```python
from build123d import *
from build123d.topology import SkipClean

# Parameters (mm, degrees)
BOSS_EXTRUDE1_DEPTH     = 3
CROQUIS1_W              = 50.575264902
CROQUIS1_H              = 364.883290788
CROQUIS1_W_2            = 121.011581191
CROQUIS1_H_2            = 356.31671178
CORTAR_EXTRUIR1_DEPTH   = 10
CROQUIS2_W              = 390
CROQUIS2_H              = 250
SALIENTE_EXTRUIR1_DEPTH = 3
CROQUIS3_W              = 60
CROQUIS3_H              = 30
CORTAR_EXTRUIR3_DEPTH   = 3
CROQUIS4_W              = 90
CROQUIS4_H              = 3
SALIENTE_EXTRUIR2_DEPTH = 3
CROQUIS5_W              = 30
CROQUIS5_H              = 30
CORTAR_EXTRUIR4_DEPTH   = 3
CROQUIS6_W              = 30
CROQUIS6_H              = 38.5
CORTAR_EXTRUIR5_DEPTH   = 3
CROQUIS7_W              = 38.5
CROQUIS7_H              = 30
CORTAR_EXTRUIR6_DEPTH   = 3
CROQUIS8_W              = 137
CROQUIS8_H              = 0.25
CORTAR_EXTRUIR7_DEPTH   = 3
CROQUIS9_W              = 0.25
CROQUIS9_H              = 68.25
CORTAR_EXTRUIR8_DEPTH   = 3
CORTAR_EXTRUIR9_DEPTH   = 3
SALIENTE_EXTRUIR3_DEPTH = 3
CROQUIS12_R             = 4
CORTAR_EXTRUIR10_DEPTH  = 3
CROQUIS13_R             = 4.25
CROQUIS13_R_2           = 3.25
SALIENTE_EXTRUIR4_DEPTH = 3
CROQUIS14_R             = 4.25
CORTAR_EXTRUIR11_DEPTH  = 3
CROQUIS15_R             = 4.25
CORTAR_EXTRUIR12_DEPTH  = 25
SALIENTE_EXTRUIR5_DEPTH = 3
CROQUIS17_R             = 1.5
CORTAR_EXTRUIR13_DEPTH  = 10
CROQUIS18_R             = 1.5
CORTAR_EXTRUIR14_DEPTH  = 30
CROQUIS19_R             = 1.5
SALIENTE_EXTRUIR6_DEPTH = 3
CROQUIS21_R             = 1.5
CORTAR_EXTRUIR15_DEPTH  = 3
SALIENTE_EXTRUIR7_DEPTH = 3
CORTAR_EXTRUIR17_DEPTH  = 10
CORTAR_EXTRUIR18_DEPTH  = 10


with BuildPart() as part:
    # Sketch1 → Boss-Extrude1 (new body)
    with BuildSketch(Plane.XY):
        Polygon((0, 0), (403.39, 0), (403.39, 241), (274.41, 359.5), (128.98, 359.5), (0, 241), align=None)
        Polygon((216.695, 223), (246.695, 223), (246.695, 253), (156.695, 253), (156.695, 223), (186.695, 223), (186.695, 219.825), (216.695, 219.825), align=None, mode=Mode.SUBTRACT)
    extrude(amount=BOSS_EXTRUDE1_DEPTH)

    # Croquis1 → Cortar-Extruir1 (cut)
    with BuildSketch(Plane.XY.offset(3)):
        with Locations((-18.592632451, 182.441645394)):
            Rectangle(CROQUIS1_W, CROQUIS1_H)
        with Locations((457.200790596, 178.15835589)):
            Rectangle(CROQUIS1_W_2, CROQUIS1_H_2)
    extrude(amount=-CORTAR_EXTRUIR1_DEPTH, mode=Mode.SUBTRACT)

    # Croquis2 → Saliente-Extruir1 (add)
    with BuildSketch(Plane.XY.offset(3)):
        with Locations((201.695, 125)):
            Rectangle(CROQUIS2_W, CROQUIS2_H)
    extrude(amount=-SALIENTE_EXTRUIR1_DEPTH)

    # Croquis3 → Cortar-Extruir3 (cut)
    with BuildSketch(Plane.XY.offset(3)):
        with Locations((201.695, 235)):
            Rectangle(CROQUIS3_W, CROQUIS3_H)
    extrude(amount=-CORTAR_EXTRUIR3_DEPTH, mode=Mode.SUBTRACT)

    # Croquis4 → Saliente-Extruir2 (add)
    with BuildSketch(Plane.XY.offset(3)):
        with Locations((201.695, 251.5)):
            Rectangle(CROQUIS4_W, CROQUIS4_H)
    extrude(amount=-SALIENTE_EXTRUIR2_DEPTH)

    # Croquis5 → Cortar-Extruir4 (cut)
    with BuildSketch(Plane.XY.offset(3)):
        with Locations((201.695, 205)):
            Rectangle(CROQUIS5_W, CROQUIS5_H)
    extrude(amount=-CORTAR_EXTRUIR4_DEPTH, mode=Mode.SUBTRACT)

    # Croquis6 → Cortar-Extruir5 (cut)
    with BuildSketch(Plane.XY.offset(3)):
        with Locations((201.695, 170.75)):
            Rectangle(CROQUIS6_W, CROQUIS6_H)
    extrude(amount=-CORTAR_EXTRUIR5_DEPTH, mode=Mode.SUBTRACT)

    # Croquis7 → Cortar-Extruir6 (cut)
    with BuildSketch(Plane.XY.offset(3)):
        with Locations((152.445, 235)):
            Rectangle(CROQUIS7_W, CROQUIS7_H)
        with Locations((250.945, 235)):
            Rectangle(CROQUIS7_W, CROQUIS7_H)
    extrude(amount=-CORTAR_EXTRUIR6_DEPTH, mode=Mode.SUBTRACT)

    # Croquis8 → Cortar-Extruir7 (cut)
    with BuildSketch(Plane.XY.offset(3)):
        with Locations((201.695, 250.125)):
            Rectangle(CROQUIS8_W, CROQUIS8_H)
        with Locations((201.695, 219.875)):
            Rectangle(CROQUIS8_W, CROQUIS8_H)
    extrude(amount=-CORTAR_EXTRUIR7_DEPTH, mode=Mode.SUBTRACT)

    # Croquis9 → Cortar-Extruir8 (cut)
    with BuildSketch(Plane.XY.offset(3)):
        with Locations((186.57, 185.625)):
            Rectangle(CROQUIS9_W, CROQUIS9_H)
        with Locations((216.82, 185.625)):
            Rectangle(CROQUIS9_W, CROQUIS9_H)
    extrude(amount=-CORTAR_EXTRUIR8_DEPTH, mode=Mode.SUBTRACT)

    # Croquis10 → Cortar-Extruir9 (cut)
    with BuildSketch(Plane.XY.offset(3)):
        Polygon((136.695, 348.165217873), (266.695, 348.165217873), (396.695, 250), (402.242964747, 389.308105161), (24.251899655, 412.117910813), (6.695, 250), align=None)
    extrude(amount=-CORTAR_EXTRUIR9_DEPTH, mode=Mode.SUBTRACT)

    # Croquis11 → Saliente-Extruir3 (add)
    with BuildSketch(Plane.XY.offset(3)):
        Polygon((51.733112384, 284.009047037), (6.695, 250), (31.650370126, 216.951653685), align=None)
        Polygon((347.889102287, 286.854166019), (396.695, 250), (356.623353442, 225.729213199), align=None)
    extrude(amount=-SALIENTE_EXTRUIR3_DEPTH)

    # Croquis12 → Cortar-Extruir10 (cut)
    with BuildSketch(Plane.XY.offset(3)):
        with Locations((21.695, 15)):
            Circle(CROQUIS12_R)
        with Locations((381.695, 15)):
            Circle(CROQUIS12_R)
        with Locations((51.695, 235)):
            Circle(CROQUIS12_R)
        with Locations((351.695, 235)):
            Circle(CROQUIS12_R)
    extrude(amount=-CORTAR_EXTRUIR10_DEPTH, mode=Mode.SUBTRACT)

    # Croquis13 → Saliente-Extruir4 (add)
    # profile 1 of 2: a face of its own
    with BuildSketch(Plane.XY.offset(3)):
        with Locations((51.695, 235)):
            Circle(CROQUIS13_R)
        with Locations((51.695, 235)):
            Circle(CROQUIS13_R_2, mode=Mode.SUBTRACT)
    # profile 2 of 2: a face of its own
    with BuildSketch(Plane.XY.offset(3)):
        with Locations((351.695, 235)):
            Circle(CROQUIS13_R)
        with Locations((351.695, 235)):
            Circle(CROQUIS13_R_2, mode=Mode.SUBTRACT)
    extrude(amount=-SALIENTE_EXTRUIR4_DEPTH)

    # Croquis14 → Cortar-Extruir11 (cut)
    with BuildSketch(Plane.XY.offset(3)):
        with Locations((201.695, 35)):
            Circle(CROQUIS14_R)
        with Locations((201.695, 123)):
            Circle(CROQUIS14_R)
    extrude(amount=-CORTAR_EXTRUIR11_DEPTH, mode=Mode.SUBTRACT)

    # Croquis15 → Cortar-Extruir12 (cut)
    with BuildSketch(Plane.XY.offset(3)):
        with Locations((201.695, 38)):
            Circle(CROQUIS15_R)
    extrude(amount=-CORTAR_EXTRUIR12_DEPTH, mode=Mode.SUBTRACT)

    # Croquis16 → Saliente-Extruir5 (add)
    with BuildSketch(Plane.XY.offset(3)):
        with BuildLine():
            ThreePointArc((205.67149343, 36.5), (201.695, 33.75), (197.71850657, 36.5))
            ThreePointArc((197.71850657, 36.5), (200.9326343, 30.818935717), (205.945, 35))
            ThreePointArc((205.945, 35), (205.876064283, 35.7623657), (205.67149343, 36.5))
        make_face()
    extrude(amount=-SALIENTE_EXTRUIR5_DEPTH)

    # Croquis17 → Cortar-Extruir13 (cut)
    with BuildSketch(Plane.XY.offset(3)):
        with Locations((146.568722662, 341.065217873)):
            Circle(CROQUIS17_R)
        with Locations((254.977292633, 341.065217873)):
            Circle(CROQUIS17_R)
        with Locations((134.589248293, 337.678282679)):
            Circle(CROQUIS17_R)
        with Locations((31.642655291, 259.941553977)):
            Circle(CROQUIS17_R)
        with Locations((268.800751707, 337.678282679)):
            Circle(CROQUIS17_R)
        with Locations((371.747344709, 259.941553977)):
            Circle(CROQUIS17_R)
    extrude(amount=-CORTAR_EXTRUIR13_DEPTH, mode=Mode.SUBTRACT)

    # Croquis18 → Cortar-Extruir14 (cut)
    with BuildSketch(Plane.XY.offset(3)):
        with Locations((144.695, 341.065217873)):
            Circle(CROQUIS18_R)
        with Locations((258.695, 341.065217873)):
            Circle(CROQUIS18_R)
    extrude(amount=-CORTAR_EXTRUIR14_DEPTH, mode=Mode.SUBTRACT)

    # Croquis19 → Saliente-Extruir6 (add)
    with BuildSketch(Plane.XY.offset(3)):
        with BuildLine():
            ThreePointArc((145.631861331, 339.893769689), (145.068722662, 341.065217873), (145.631861331, 342.236666056))
            ThreePointArc((145.631861331, 342.236666056), (143.195, 341.065217873), (145.631861331, 339.893769689))
        make_face()
        with Locations((254.977292633, 341.065217873)):
            Circle(CROQUIS19_R)
    extrude(amount=-SALIENTE_EXTRUIR6_DEPTH)

    # Croquis21 → Cortar-Extruir15 (cut)
    with BuildSketch(Plane.XY.offset(3)):
        with Locations((144.695, 341.065217873)):
            Circle(CROQUIS21_R)
    extrude(amount=-CORTAR_EXTRUIR15_DEPTH, mode=Mode.SUBTRACT)

    # Croquis22 → Saliente-Extruir7 (add)
    with BuildSketch(Plane.XY.offset(3)):
        with BuildLine():
            ThreePointArc((145.631861331, 342.236666056), (146.046904582, 341.715105557), (146.195, 341.065217873))
            ThreePointArc((146.195, 341.065217873), (146.046904582, 340.415330189), (145.631861331, 339.893769689))
            ThreePointArc((145.631861331, 339.893769689), (147.218610346, 339.713313291), (148.068722662, 341.065217873))
            ThreePointArc((148.068722662, 341.065217873), (147.218610346, 342.417122454), (145.631861331, 342.236666056))
        make_face()
    extrude(amount=-SALIENTE_EXTRUIR7_DEPTH)

    # Croquis23 → Cortar-Extruir17 (cut)
    with BuildSketch(Plane.XY.offset(3)):
        with BuildLine():
            ThreePointArc((163.945, 204.75), (169.248300859, 202.553300859), (171.445, 197.25))
            Line((171.445, 197.25), (171.445, 171.4))
            Line((171.445, 171.4), (153.095, 171.4))
            Line((153.095, 171.4), (153.095, 204.75))
            Line((153.095, 204.75), (163.945, 204.75))
        make_face()
        with BuildLine():
            Line((250.295, 204.75), (239.445, 204.75))
            ThreePointArc((239.445, 204.75), (234.141699141, 202.553300859), (231.945, 197.25))
            Line((231.945, 197.25), (231.945, 171.4))
            Line((231.945, 171.4), (250.295, 171.4))
            Line((250.295, 171.4), (250.295, 204.75))
        make_face()
    extrude(amount=-CORTAR_EXTRUIR17_DEPTH, mode=Mode.SUBTRACT)

    # Croquis25 → Cortar-Extruir18 (cut)
    with SkipClean():  # the faces are left unmerged after this step: merging them gives an invalid solid
        with BuildSketch(Plane.XY.offset(3)):
            Polygon((195.695, 38), (195.695, 30), (207.695, 30), (207.695, 38), (207.695, 68), (195.695, 68), align=None)
        extrude(amount=-CORTAR_EXTRUIR18_DEPTH, mode=Mode.SUBTRACT)


solid = part.part
```
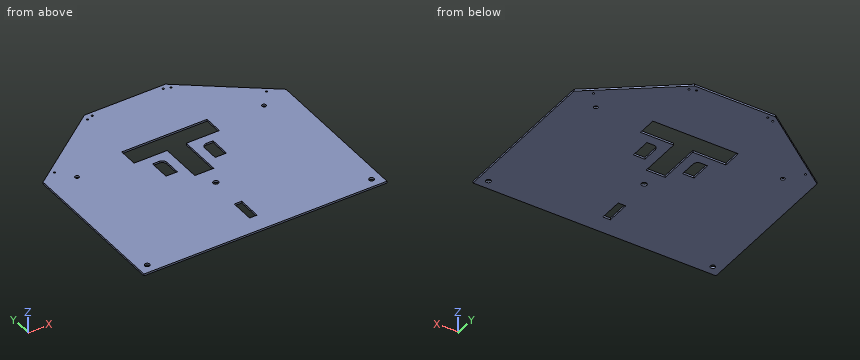
The model under review builds one solid part; all positions refer to its coordinate system, in mm. Round coordinates to 2 decimals unless told otherwise and drop trailing zeros. Loops run counter-clockwise (first coordinate to the right, second up) from the corner with the lowest first, then second, coordinate; pieces in that order, holes last. Notation, with made-up numbers: (-11, -27.75) - (4, -27.75) arc R21 cw to (4, -12.75) - close; hole circle Ø7 at (9, 89). An arc over 180 degrees is marked (long way). Write each question's results on one line, items separated by ' | '. Start each with the question number.
Q1. Wall thickness on line 1 along Y through (x, z) = (158, 1); line 2 along Y through (x, z) = (256, 2.05); line 3 along X through (y, z) = (249.5, 1.1) (3 decimals): over which ranges is each line inside the solid? List them lowest first. Write a range as [from, to].
Q2. Insertion check: P1, Ø2.5, axis at x = 31.64, y = 259.94, coming from the -Z side. The pin has a flat end and moves straight along its axis. Give the tip position at first contact, or say it passes through.
Q3. Take a section at B-B on y = 57. Give the boundary of the cut face in (x, z) (3 decimals).
Q4. Take a section at A-A on y = 123. Give the boundary of the cut face in (x, z) (3 decimals).
Q5. Take a section at D-D on z = 0.75. Give the number of separate pieces and of enclosed holes in the cut face, plus the area to 3 significant figures.
Q6. Take a section at C-C on x = 363.5. Give the boundary of the cut face in (y, z).
Data:
1) line 1: y = [0, 171.4], [204.75, 219.75], [250.25, 348.17] | line 2: y = [0, 219.75], [250.25, 348.17] | line 3: x = [6.695, 133.195], [270.195, 396.695]
2) P1: passes through
3) outline: (6.695, 0) - (195.695, 0) - (195.695, 3) - (6.695, 3) - close; (207.695, 0) - (396.695, 0) - (396.695, 3) - (207.695, 3) - close
4) outline: (6.695, 0) - (197.445, 0) - (197.445, 3) - (6.695, 3) - close; (205.945, 0) - (396.695, 0) - (396.695, 3) - (205.945, 3) - close
5) separate pieces: 1 | enclosed holes: 15 | area: 115,000 mm²
6) outline: (0, 0) - (275.07, 0) - (275.07, 3) - (0, 3) - close
